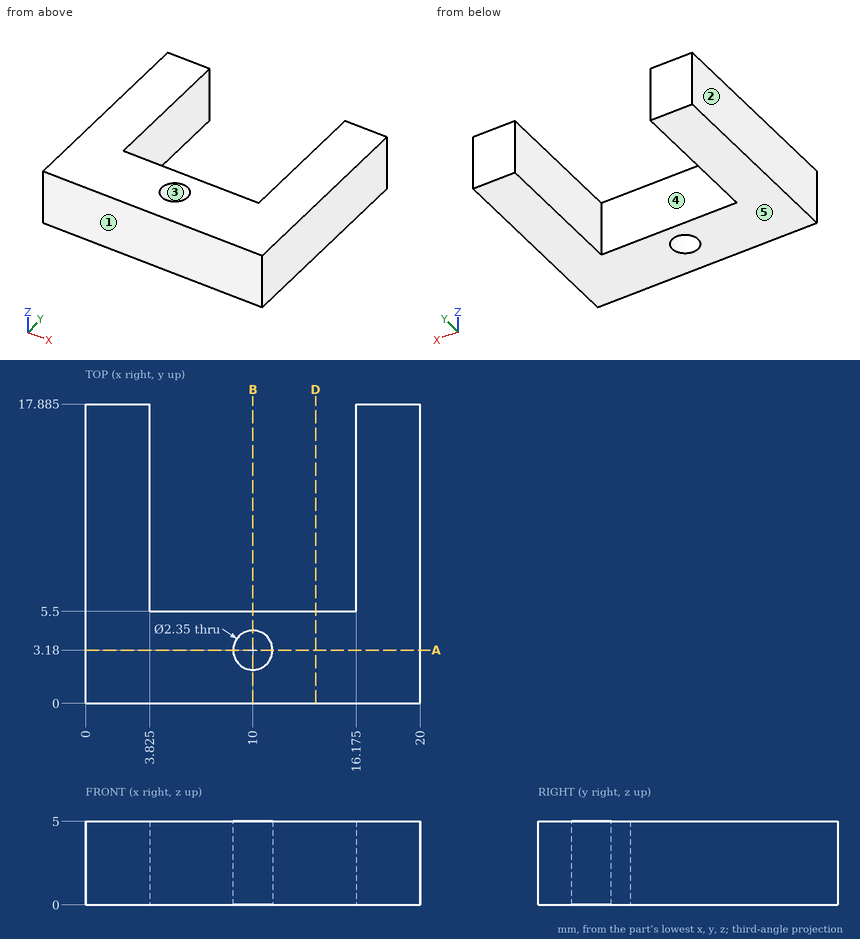
Can you work these out from the drawing? Everything is in mm from the part's minimum corner. A direction names the side the tool comes from. Coordinates: 2 decimals unless noted, no trailing zeros. Write each loop counter-clockwise with the first axis right and the second up, starting at its lowest first coordinate (ties: lowest second). Pieces come first, ordered by that corner, then holes. Notation, with made-up numbers: (77.25, 43.25) -> (119.25, 43.25) arc R17 cw to (119.25, 57.25) -> close; hole circle Ø6 at (72.5, 69). An arc over 180 degrees is marked (long way). Return JSON: item names as keys, results as strings.
(1) Imagine slicing it at B-B, the plane x = 10. Please give me the cut outline in (y, z) (1 decimal).
Numbers:
{"outline": "(0, 0) -> (2, 0) -> (2, 5) -> (0, 5) -> close; (4.4, 0) -> (5.5, 0) -> (5.5, 5) -> (4.4, 5) -> close"}
(2) We'd pull the mould along X, two halves only. Please class the marked faces 1, 2 and 3: +X half, -X half, draft (parallel to the pull), parting line (faces both ways), or undercut.
Numbers:
{"face 1": "draft", "face 2": "-X half", "face 3": "undercut"}
(3) I'm going to push a flat-ended pin straight in: pin 1 (1.4 mm diameter, centred on x = 10, y = 3.18, fed in from +Z). Where does the tip first touch, or does it pass through?
Numbers:
{"pin 1": "passes through"}
(4) Imagine slicing it at D-D, the plane x = 13.75. Please give me the cut outline in (y, z).
Numbers:
{"outline": "(0, 0) -> (5.5, 0) -> (5.5, 5) -> (0, 5) -> close"}
(5) Which directions (+Z, -Z, +X, -X, +Y, -Y) give clear straight access to the entire face, cutting with the end or side of a thin tool? Please do the marked faces 4 and 5.
Numbers:
{"face 4": "+Z, -Z, +Y", "face 5": "-Z, +X, -X, +Y, -Y"}
(6) I need wall thicknesses on L1, parallel to X at y = 3.18, z = 1.3 (1 decimal); L2, parallel to X at y = 8, z = 2.7 (1 decimal); L3, parallel to Y at x = 10, z = 2.9 (1 decimal). Which ranges of each line are inside material? Lowest first, please.
Numbers:
{"L1": "x = 0 to 8.8, 11.2 to 20", "L2": "x = 0 to 3.8, 16.2 to 20", "L3": "y = 0 to 2, 4.4 to 5.5"}
(7) Imagine slicing it at A-A, the plane y = 3.18. Please give me the cut outline in (x, z) (1 decimal).
Numbers:
{"outline": "(0, 0) -> (8.8, 0) -> (8.8, 5) -> (0, 5) -> close; (11.2, 0) -> (20, 0) -> (20, 5) -> (11.2, 5) -> close"}
